Geometry: final body of the model. Coordinates: model frame, mm. Give positions to 0.01 mm unless a question says otherwise; leave off trailing zeros. Order: outer loops, then holes, each group sorted by start corner. A loop starts at its lowest first (then second) coordinate and runs counter-clockwise, first axis right, second up. Notation, with made-up numbers: M 30,20.25 L 64,20.25 A23 cw 64,37.25 Z; hole C 9,36 d6. An arc over 180 degrees is marked long. One line per item, written item: value. Start each with the question number.
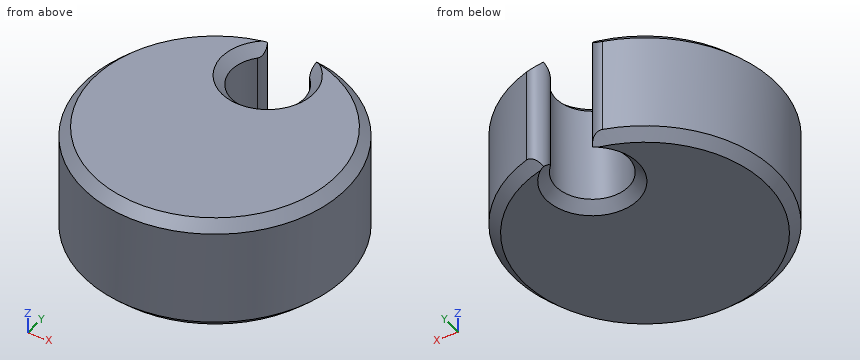
Autodesk Inventor part; units mm, degrees
ref_plane "YZ Plane" through (0, 0, 0) normal (1, 0, 0) x (0, 1, 0)
ref_plane "XZ Plane" through (0, 0, 0) normal (0, 1, 0) x (-1, 0, 0)
ref_plane "XY Plane" through (0, 0, 0) normal (0, 0, 1) x (1, 0, 0)
sketch "Sketch1" plane through (0, 0, 0) normal (0, 0, 1) x (1, 0, 0)
  circle A0 centre (0, 0) radius 4
  dimension "d0" = 8
extrude "Extrusion1" add sketch "Sketch1" along normal blind 3.5
sketch "Sketch4" plane through (0, 0, 0) normal (0, 0, -1) x (-1, 0, 0)
  line L0 (0, 0) -> (0, 2.5)
  circle A0 centre (0, 2.5) radius 1.1
  dimension "d9" = 2.5
  dimension "d10" = 2.2
extrude "Extrusion3" cut sketch "Sketch4" against normal through all
chamfer "Chamfer1" distance 0.3 angle 45 4 edges at (-4, 0, 3.5) (-4, 0, 0) (1.1, 2.5, 0) (1.1, 2.5, 3.5)
sketch "Sketch5" plane through (0, 0, 3.5) normal (0, 0, 1) x (1, 0, 0)
  line L0 (-0.4, 4.2659) -> (0.4, 4.2659)
  line L1 (0.4, 4.2659) -> (0.4, 2.9071)
  line L2 (0.4, 2.9071) -> (-0.4, 2.9071)
  line L3 (-0.4, 2.9071) -> (-0.4, 4.2659)
  circle A0 centre (0, 2.5) radius 1.1 construction
  point P0 (0, 0)
  dimension "d16" = 0.4
  dimension "d17" = 0.4
extrude "Extrusion4" cut sketch "Sketch5" against normal through all
fillet "Fillet1" radius 0.35 4 edges at (-0.4, 3.5247, 1.75) (-0.4, 3.9799, 1.75) (0.4, 3.5247, 1.75) (0.4, 3.9799, 1.75)
equation "\"d17\" = d16"
properties part number "CamShaft"
Q1. Section query A-A on x = 0. Return loops of the section in (y, z), and give its area (3 significant figures).
Q2. Contact query for flat-ended pins moving along their axis: pin 1 (1 mm diameter, centred on x = 1.5, z = 3, fed in from +Y); pin 2 (1.5 mm diameter, centred on y = -1.5, z = 2.5, fed in from +X); pin 3 (1.5 mm diameter, centred on x = 2.5, z = 0.5, fed in from -Y); pin 4 (2.5 mm diameter, centred on x = 0, y = 2.5, fed in from +Z). Output: stop coordinate, or through.
Q3. Ray query, line 1 along Y through (x, z) = (0, 2.3); line 2 along X through (y, z) = (2.75, 2.8); line 3 along X through (y, z) = (2.5, 2.4). Return the intervals inside material, ascending. Write a range as [from, to].
Q4. Section query B-B on z = 2.35. Return loops of the section in (x, y), and give its area (3 significant figures).
Results below:
1. outline: M -4,0.3 L -3.7,0 L 1.1,0 L 1.4,0.3 L 1.4,3.2 L 1.1,3.5 L -3.7,3.5 L -4,3.2 Z
1. area: 18.7 mm2
2. pin 1: y = 3.84
2. pin 2: x = 3.93
2. pin 3: y = -3.6
2. pin 4: z = 3.35
3. line 1: [-4, 1.4]
3. line 2: [-2.9, -1.07], [1.07, 2.9]
3. line 3: [-3.12, -1.1], [1.1, 3.12]
4. outline: M -1.16,3.83 A4 ccw long 1.16,3.83 A0.35 ccw 0.8,3.25 A1.1 cw long -0.8,3.25 A0.35 ccw Z
4. area: 45.7 mm2
